Part model, mm, in its own coordinate system. A direction names the side the tool comes from. Coordinates: 2 decimals unless noted, no trailing zeros. Loops run counter-clockwise (first coordinate to the right, second up) from the corner with the lowest first, then second, coordinate; pieces in that order, holes last. Notation, with made-up numbers: (-23, -11.75) - (-16, -11.75) arc R10 cw to (-16, 0.25) - close; hole circle Ø11 at (-20, 49). An arc over 180 degrees is marked (long way). Use a Markdown table: item, result. Add a question column.
1. Band-saw the part on B-B, the plane x = 203. Give the cut face in (y, z).
2. 3-axis set-ups, long thin cutter, end or side, ignore diameter. For faces 5 (the flat face through (-300, -1, 1)), 6 (the flat face through (4, -16, 150.5)): which of +Z, -Z, +X, -X, +Y, -Y reach the whole face in a straight line?
3. Wall check: probe 1 along Z at (x, y) = (-96, -16.75); probe 2 along Y at (x, z) = (-7, -24.5). Give the ranges that are in metal, low to high. Write a range as [from, to].
4. Drop flat-ended pins along their axis: pin 1 (12 mm diameter, centred on x = -27.5, z = -62, fed in from -Y); pin 2 (6 mm diameter, centred on y = -6.5, z = 57, fed in from +X); pin 3 (2 mm diameter, centred on x = -150, z = -33, fed in from +Y). Give the stop position or say it passes through.
5. Pull direction Z, two halves, no side cores. Call faces 1 (the flat face through (300, -1, 1)), 2 (the flat face through (-4, -13, -152)), 3 (the flat face through (-4, -13, -150.5)), 4 (the flat face through (4, -16, 152)): pulls with the +Z half, pulls with the -Z half, needs draft (parallel to the pull), parting line crosses it, or undercut.
6. Band-saw the part on A-A, the plane y = -24.5. Count the separate pieces of the cut face and the enclosed holes in it, plus the area to 3 significant figures.
7. Band-saw the part on C-C, the plane z = 8. Give the cut face in (x, y).
from build123d import *

# Parameters (mm, degrees)
SKETCH_1_W                         = 600
SKETCH_1_H                         = 304
SM_BASE_FLANGE_1_DEPTH             = 1.5
SM_EDGE_FLANGE_1_STRIP_W           = 7.4732
SM_EDGE_FLANGE_1_STRIP_H           = 1.5
SM_EDGE_FLANGE_1_STRIP_CUT_DEPTH   = 600
SM_EDGE_FLANGE_1_STRIP_2_W         = 7.4732
SM_EDGE_FLANGE_1_STRIP_2_H         = 1.5
SM_EDGE_FLANGE_1_STRIP_CUT_2_DEPTH = 600
SM_EDGE_FLANGE_1_DEPTH             = 600
SM_EDGE_FLANGE_1_BEND_DEPTH        = 600
CUT_EXTRUDE_1_DEPTH                = 429.154177838
PATTERN_LINEAR_1_COUNT             = 3
PATTERN_LINEAR_1_PITCH             = 255


# Sheet-metal steps are written as plain solids
with BuildPart() as part:
    # Sketch 1 → 基体-法兰1 (new body)
    with BuildSketch(Plane(origin=(0, 0, 0), x_dir=(1, 0, 0), z_dir=(0, 1, 0))):
        Rectangle(SKETCH_1_W, SKETCH_1_H)
    extrude(amount=-SM_BASE_FLANGE_1_DEPTH)

    # 边线-法兰1 strip (across the edge) → 边线-法兰1 strip cut (cut)
    with BuildSketch(Plane(origin=(300, -1.5, 152), x_dir=(0, 0, -1), z_dir=(-1, 0, 0))):
        with Locations((-1.5, -0.75)):
            Rectangle(SM_EDGE_FLANGE_1_STRIP_W, SM_EDGE_FLANGE_1_STRIP_H)
    extrude(amount=SM_EDGE_FLANGE_1_STRIP_CUT_DEPTH, mode=Mode.SUBTRACT)

    # 边线-法兰1 strip 2 (across the edge) → 边线-法兰1 strip cut 2 (cut)
    with BuildSketch(Plane(origin=(-300, -1.5, -152), x_dir=(0, 0, 1), z_dir=(1, 0, 0))):
        with Locations((-1.5, -0.75)):
            Rectangle(SM_EDGE_FLANGE_1_STRIP_2_W, SM_EDGE_FLANGE_1_STRIP_2_H)
    extrude(amount=SM_EDGE_FLANGE_1_STRIP_CUT_2_DEPTH, mode=Mode.SUBTRACT)

    # 边线-法兰1 section (across the edge) → 边线-法兰1 (add)
    with BuildSketch(Plane(origin=(300, -1.5, 152), x_dir=(0, 0, -1), z_dir=(-1, 0, 0))):
        with BuildLine():
            Line((0, 0.7366), (0, 28.5))
            Line((0, 28.5), (1.5, 28.5))
            Line((1.5, 28.5), (1.5, 0.7366))
            ThreePointArc((1.5, 0.7366), (1.715745145, 0.215745145), (2.2366, 0))
            Line((2.2366, 0), (2.2366, -1.5))
            ThreePointArc((2.2366, -1.5), (0.655084973, -0.844915027), (0, 0.7366))
        make_face()
    extrude(amount=SM_EDGE_FLANGE_1_DEPTH)

    # 边线-法兰1 section 2 (across the edge) → 边线-法兰1 bend (add)
    with BuildSketch(Plane(origin=(-300, -1.5, -152), x_dir=(0, 0, 1), z_dir=(1, 0, 0))):
        with BuildLine():
            Line((0, 0.7366), (0, 28.5))
            Line((0, 28.5), (1.5, 28.5))
            Line((1.5, 28.5), (1.5, 0.7366))
            ThreePointArc((1.5, 0.7366), (1.715745145, 0.215745145), (2.2366, 0))
            Line((2.2366, 0), (2.2366, -1.5))
            ThreePointArc((2.2366, -1.5), (0.655084973, -0.844915027), (0, 0.7366))
        make_face()
    extrude(amount=SM_EDGE_FLANGE_1_BEND_DEPTH)

    # 草图12 → 切除-拉伸1 (cut, through all)
    with BuildSketch(Plane(origin=(0, 0, -152), x_dir=(-1, 0, 0), z_dir=(0, 0, -1))):
        with BuildLine():
            Line((-254.5, -30), (-254.5, -20))
            ThreePointArc((-254.5, -20), (-250, -15.5), (-245.5, -20))
            Line((-245.5, -20), (-245.5, -30))
            ThreePointArc((-245.5, -30), (-250, -34.5), (-254.5, -30))
        make_face()
    cut_extrude_1 = extrude(amount=-CUT_EXTRUDE_1_DEPTH, mode=Mode.SUBTRACT)

    # 阵列(线性)1: 切除-拉伸1 ×3
    with Locations(*[(-i * PATTERN_LINEAR_1_PITCH, 0, 0) for i in range(1, PATTERN_LINEAR_1_COUNT)]):
        add(cut_extrude_1, mode=Mode.SUBTRACT)


solid = part.part
Geometry check:
| question | item | result |
|---|---|---|
| 1 | outline | (-30, -152) - (-2.24, -152) arc R2.24 ccw to (0, -149.76) - (0, 149.76) arc R2.24 ccw to (-2.24, 152) - (-30, 152) - (-30, 150.5) - (-2.24, 150.5) arc R0.74 cw to (-1.5, 149.76) - (-1.5, -149.76) arc R0.74 cw to (-2.24, -150.5) - (-30, -150.5) - close |
| 2 | face 5 | +Z, -Z, -X, +Y, -Y |
| 2 | face 6 | +X, -X, -Y |
| 3 | probe 1 | z = [-152, -150.5], [150.5, 152] |
| 3 | probe 2 | y = [-1.5, 0] |
| 4 | pin 1 | stops at y = -1.5 |
| 4 | pin 2 | passes through |
| 4 | pin 3 | stops at y = 0 |
| 5 | face 1 | needs draft |
| 5 | face 2 | pulls with the -Z half |
| 5 | face 3 | undercut |
| 5 | face 4 | pulls with the +Z half |
| 6 | separate pieces | 8 |
| 6 | enclosed holes | 0 |
| 6 | area | 1,720 mm^2 |
| 7 | outline | (-300, -1.5) - (300, -1.5) - (300, 0) - (-300, 0) - close |
